CAD build for the part. Positions are in the model's coordinates, mm. A direction names the side the tool comes from. Round coordinates to 2 decimals unless told otherwise and drop trailing zeros. Order: outer loops, then holes, each group sorted by start corner. A loop starts at its lowest first (then second) coordinate and runs counter-clockwise, first axis right, second up. Notation, with made-up numbers: M -32.75,-16.75 L -20.75,-16.75 A20 cw -20.75,10.25 Z; hole C 86.5,-15.75 d4. An arc over 180 degrees is marked long. Answer as CSV lines item,"result". Start each with the question number.
```python
from build123d import *

# Parameters (mm, degrees)
SKETCH1_W           = 152.4
SKETCH1_H           = 165.1
BOSS_EXTRUDE1_DEPTH = 4.7625
CUT_EXTRUDE1_DEPTH  = 5.7625
SKETCH3_R           = 3.175
CUT_EXTRUDE2_DEPTH  = 5.7625


with BuildPart() as part:
    # Sketch1 → Boss-Extrude1 (new body)
    with BuildSketch(Plane(origin=(0, 0, 0), x_dir=(0, 0, -1), z_dir=(1, 0, 0))):
        with Locations((76.2, 0)):
            Rectangle(SKETCH1_W, SKETCH1_H)
    extrude(amount=BOSS_EXTRUDE1_DEPTH)

    # Sketch2 → Cut-Extrude1 (cut, through all)
    with BuildSketch(Plane.ZY):
        with BuildLine():
            Line((-107.95, 25.4), (-107.95, -25.4))
            ThreePointArc((-107.95, -25.4), (-106.090128061, -29.890128061), (-101.6, -31.75))
            Line((-101.6, -31.75), (-50.8, -31.75))
            ThreePointArc((-50.8, -31.75), (-46.309871939, -29.890128061), (-44.45, -25.4))
            Line((-44.45, -25.4), (-44.45, 25.4))
            ThreePointArc((-44.45, 25.4), (-46.309871939, 29.890128061), (-50.8, 31.75))
            Line((-50.8, 31.75), (-101.6, 31.75))
            ThreePointArc((-101.6, 31.75), (-106.090128061, 29.890128061), (-107.95, 25.4))
        make_face()
    extrude(amount=-CUT_EXTRUDE1_DEPTH, mode=Mode.SUBTRACT)

    # Sketch3 → Cut-Extrude2 (cut, through all)
    with BuildSketch(Plane.ZY):
        with Locations((-60.325, 69.85)):
            Circle(SKETCH3_R)
        with Locations((-92.075, 69.85)):
            Circle(SKETCH3_R)
        with Locations((-92.075, -69.85)):
            Circle(SKETCH3_R)
        with Locations((-60.325, -69.85)):
            Circle(SKETCH3_R)
    extrude(amount=-CUT_EXTRUDE2_DEPTH, mode=Mode.SUBTRACT)


solid = part.part
```
Q1. Band-saw the part on D-D, the plane x = 1.6. Write the cut outline in (y, z) (3 decimals), then the cut area to 3 significant figures.
Q2. Band-saw the part on A-A, the plane z = -80. Write the cut outline in (x, y).
Q3. Band-saw the part on B-B, the plane y = -69.85. Write the cut outline in (x, z).
Q4. Probe line 1 along Z through (x, y) = (1, 71.5); line 2 along Y through (x, z) = (1.1, -70.5); line 3 along Z through (x, y) = (1.9, -2.5). List the from-to ranges inside material, lowest first. Write a range as from..to.
Q5. Mould opens along Y. For faces 1 (the cylindrical face through (2.35, 29.84, -46.26)), 2 (the flat face through (2, -1, -152.4)), 3 (the flat face through (2, 82.55, -75)) say: +Y half, -Y half, draft (parallel to the pull), parting line (faces both ways), or undercut.
Q6. Band-saw the part on C-C, the plane y = -16. Write the cut outline in (x, z).
Q7. Tool access for faces 4 (the flat face through (2, -82.55, -75)), 5 (the flat face through (2, 0, -44.45)): list every direction of +Z, -Z, +X, -X, +Y, -Y with a clear straight run to the whole face (end or side of a thin tool).
Answer:
1,outline,"M -82.55,-152.4 L 82.55,-152.4 L 82.55,0 L -82.55,0 Z; hole C -69.85,-92.075 d6.35; hole C -69.85,-60.325 d6.35; hole M -31.75,-101.6 A6.35 ccw -25.4,-107.95 L 25.4,-107.95 A6.35 ccw 31.75,-101.6 L 31.75,-50.8 A6.35 ccw 25.4,-44.45 L -25.4,-44.45 A6.35 ccw -31.75,-50.8 Z; hole C 69.85,-92.075 d6.35; hole C 69.85,-60.325 d6.35"
1,area,"21,000 mm^2"
2,outline,"M 0,-82.55 L 4.76,-82.55 L 4.76,-31.75 L 0,-31.75 Z; M 0,31.75 L 4.76,31.75 L 4.76,82.55 L 0,82.55 Z"
3,outline,"M 0,-152.4 L 4.76,-152.4 L 4.76,-95.25 L 0,-95.25 Z; M 0,-88.9 L 4.76,-88.9 L 4.76,-63.5 L 0,-63.5 Z; M 0,-57.15 L 4.76,-57.15 L 4.76,0 L 0,0 Z"
4,line 1,"z = -152.4..-94.79, -89.36..-63.04, -57.61..0"
4,line 2,"y = -82.55..-31.75, 31.75..82.55"
4,line 3,"z = -152.4..-107.95, -44.45..0"
5,face 1,"undercut"
5,face 2,"draft"
5,face 3,"+Y half"
6,outline,"M 0,-152.4 L 4.76,-152.4 L 4.76,-107.95 L 0,-107.95 Z; M 0,-44.45 L 4.76,-44.45 L 4.76,0 L 0,0 Z"
7,face 4,"+Z, -Z, +X, -X, -Y"
7,face 5,"+X, -X"
